CAD build for the part. Positions are in the model's coordinates, mm. A direction names the side the tool comes from. Give positions to 0.01 mm unless a question says otherwise; leave off trailing zeros. Order: outer loops, then holes, each group sorted by start corner. A loop starts at its lowest first (then second) coordinate and runs counter-clockwise, first axis right, second up. Notation, with made-up numbers: (36.5, 58.5) -> (79.5, 58.5) arc R30 cw to (79.5, 93.5) -> close; hole circle Ø1 at (46, -21). An arc over 180 degrees is marked (long way). Answer as CSV lines item,"result".
```python
from build123d import *

# Parameters (mm, degrees)
F1_DEPTH = 80
F2_W     = 16
F2_H     = 40
F3_DEPTH = 24.001


with BuildPart() as f1:
    # F0 (on Top) → F1 (new body)
    with BuildSketch(Plane.XY):
        Polygon((20, 0), (0, 0), (0, -4), (20, -4), (20, -44), (0, -44), (0, -48), (20, -48), (20, -64), (24, -64), (24, 16), (20, 16), align=None)
    extrude(amount=F1_DEPTH)

    # F2 (on face) → F3 (cut, through all)
    with BuildSketch(Plane.YZ.offset(24)):
        with Locations((8, 40)):
            Rectangle(F2_W, F2_H)
        with Locations((-56, 40)):
            Rectangle(F2_W, F2_H)
    extrude(amount=-F3_DEPTH, mode=Mode.SUBTRACT)


solid = f1.part
```
1) Pin check, flat tips, straight feed: P1, Ø5, axis at y = -59, z = 73.5, coming from the -X side; P2, Ø5, axis at x = 18, z = 9, coming from the +Y side; P3, Ø1.5, axis at x = 5, z = 65, coming from the +Y side; P4, Ø8, axis at x = 20.5, z = 48.5, coming from the -Y side. Stop position of each tip, or through.
Data:
P1,"stops at x = 20"
P2,"stops at y = 16"
P3,"stops at y = 0"
P4,"stops at y = -48"
2) Band-saw the part on C-C, the plane z = 10.5. Write the cut outline in (x, y), then the cut area to 3 significant figures.
Data:
outline,"(0, -48) -> (20, -48) -> (20, -64) -> (24, -64) -> (24, 16) -> (20, 16) -> (20, 0) -> (0, 0) -> (0, -4) -> (20, -4) -> (20, -44) -> (0, -44) -> close"
area,"480 mm2"
3) Band-saw the part on A-A, the plane x = 10. Write the cut outline in (y, z).
Data:
outline,"(-48, 0) -> (-44, 0) -> (-44, 80) -> (-48, 80) -> close; (-4, 0) -> (0, 0) -> (0, 80) -> (-4, 80) -> close"
4) Band-saw the part on B-B, the plane y = -57.5. Write the cut outline in (x, z).
Data:
outline,"(20, 0) -> (24, 0) -> (24, 20) -> (20, 20) -> close; (20, 60) -> (24, 60) -> (24, 80) -> (20, 80) -> close"
5) Pull direction Y, two halves, no side cores. Call faces 1 (the flat face through (10, -4, 39)), 2 (the flat face through (0, -46, 39)), 3 (the flat face through (22, -64, 70)): pulls with the +Y half, pulls with the -Y half, needs draft (parallel to the pull), parting line crosses it, or undercut.
Data:
face 1,"undercut"
face 2,"needs draft"
face 3,"pulls with the -Y half"
6) Band-saw the part on D-D, the plane y = -38. Write the cut outline in (x, z), then the cut area to 3 significant figures.
Data:
outline,"(20, 0) -> (24, 0) -> (24, 80) -> (20, 80) -> close"
area,"320 mm2"
7) Which spindle directions (+Z, -Z, +X, -X, +Y, -Y) get a long thin tool onto all of the face, cutting with end or side? Do faces 4 (the flat face through (22, 8, 20)), 5 (the flat face through (10, -44, 39)), 6 (the flat face through (22, -56, 60)). Say none if no direction does.
Data:
face 4,"+X, -X, +Y"
face 5,"+Z, -Z, -X"
face 6,"+X, -X, -Y"
8) Wall check: line 1 along Y through (x, z) = (16.5, 24.5); line 2 along Y through (x, z) = (20.25, 47); line 3 along X through (y, z) = (-6.5, 26). Give the ranges that are in metal, low to high. Write a range as [from, to].
Data:
line 1,"y = [-48, -44], [-4, 0]"
line 2,"y = [-48, 0]"
line 3,"x = [20, 24]"
